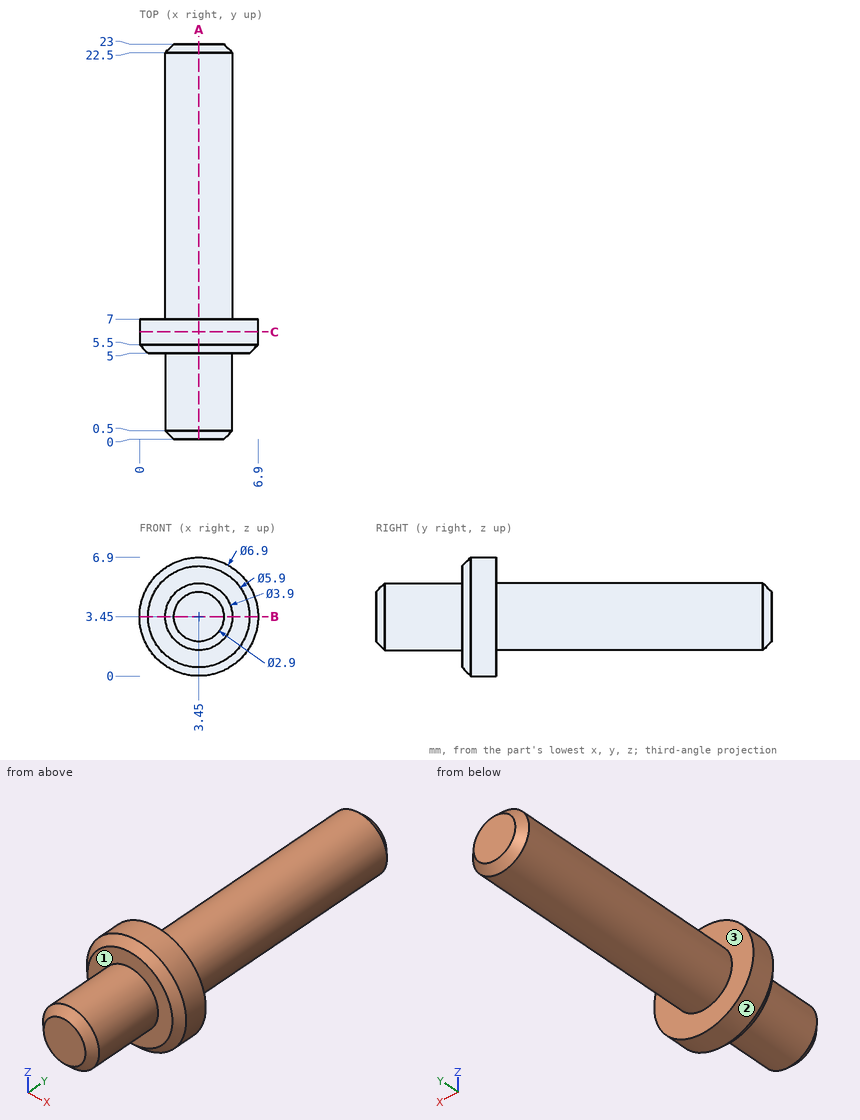
Study the drawing (mm; zero at the part's minimum x, y, z) and answer. A direction names the side the tool comes from. Round coordinates to 2 decimals unless told otherwise and drop trailing zeros. Write each loop counter-clockwise with the first axis right and the second up, starting at its lowest first coordinate (ties: lowest second). Pieces come first, ordered by that corner, then holes.
1) A cutting plane is placed at C-C on y = 6.25. Determine the outline of the cut face in (x, z).
2) A cutting plane is placed at A-A on x = 3.45. Determine the outline of the cut face in (y, z).
3) Flat-ended cylindrical pins translate along their axes: P1, Ø4, axis at y = 17.5, z = 3, coming from the +X side; P2, Ø1, axis at x = 5.5, z = 1, coming from the -Y side; P3, Ø1.5, axis at y = 3, z = 5.5, coming from the -X side. Find the tip coordinate at first contact, or state that the pin passes through.
4) Which of the six approach directions +Z, -Z, +X, -X, +Y, -Y give full straight-line access (tool end or side, diameter ignored) to the marked faces 1, 2 and 3?
5) A cutting plane is placed at B-B on z = 3.45. Determine the outline of the cut face in (x, y), and give its area (4 significant figures).
6) Consider probe 1 along Y at (x, z) = (6.25, 3.75); probe 2 along X at (y, z) = (8, 3.5). Determine where each line is inside the solid, lowest interval first.
Entries:
1. outline: circle Ø6.9 at (3.45, 3.45)
2. outline: (0, 2) - (0.5, 1.5) - (5, 1.5) - (5, 0.5) - (5.5, 0) - (7, 0) - (7, 1.5) - (22.5, 1.5) - (23, 2) - (23, 4.9) - (22.5, 5.4) - (7, 5.4) - (7, 6.9) - (5.5, 6.9) - (5, 6.4) - (5, 5.4) - (0.5, 5.4) - (0, 4.9) - close
3. P1: stops at x = 5.4
3. P2: stops at y = 5
3. P3: stops at x = 2
4. face 1: -Y
4. face 2: +Y, -Y
4. face 3: +Y
5. outline: (0, 5.5) - (0.5, 5) - (1.5, 5) - (1.5, 0.5) - (2, 0) - (4.9, 0) - (5.4, 0.5) - (5.4, 5) - (6.4, 5) - (6.9, 5.5) - (6.9, 7) - (5.4, 7) - (5.4, 22.5) - (4.9, 23) - (2, 23) - (1.5, 22.5) - (1.5, 7) - (0, 7) - close
5. area: 94.95 mm2
6. probe 1: y = 5 to 7
6. probe 2: x = 1.5 to 5.4
